Geometry: final body of the model. Coordinates: model frame, mm. A direction names the side the tool comes from. Coordinates: 2 decimals unless noted, no trailing zeros. Order: outer loops, then holes, each group sorted by start corner. A loop starts at its lowest first (then second) coordinate and runs counter-clockwise, first axis right, second up. Notation, with made-up numbers: M -28.75,46.5 L 10.25,46.5 A27 cw 10.25,64.5 Z; hole C -26.75,7 d2. An arc over 180 degrees is marked long. Use CSV: the item, a comma, the result in double quotes. Start each with the question number.
1. Material intervals for line 1 (X direction, y = -54.5, z = 7); line 2 (X direction, y = -17, z = 2.25); line 3 (Y direction, x = 32, z = 4.5), sorted ascending.
2. Section query D-D on x = 22. Return the cut outline in (y, z), and give its area (3 significant figures).
3. Section query C-C on z = 2.25. Return the cut outline in (x, y) (3 decimals), and give its area (3 significant figures).
4. Set-up query: faces 4 (the flat face through (-31.82, 37.9, 2.46)), 5 (the flat face through (65, 64, 15)), 6 (the flat face through (15, -24, 2)), 7 (the flat face through (-15, -23, 2)). Return all of +Z, -Z, +X, -X, +Y, -Y with unobstructed straight access to the full face (end or side cutting, diameter ignored); none if empty.
5. First-contact query: P1, Ø8, axis at y = 25.5, z = 7, coming from the +X side; P2, Ø1.5, axis at x = 38.5, z = 2, coming from the +Y side; P3, Ø2.5, axis at y = -23, z = 2.5, coming from the -X side. Flat tips, straight axial feed; report the tip coordinate or a pass-through.
6. Section query A-A on z = 9.25. Return the cut outline in (x, y) (3 decimals).
7. Section query B-B on y = 60.5. Return the cut outline in (x, z).
8. Pull-direction query (Y, two-part tool) for faces 1 (the cylindrical face through (0.061, 2.777, 2.535)), 2 (the flat face through (62, -59, 15)), 3 (the flat face through (42.415, 32.636, 2.465)); classes: pulls with the +Y half, pulls with the -Y half, needs draft (parallel to the pull), parting line crosses it, or undercut.
from build123d import *

# Parameters (mm, degrees)
F1_DEPTH = 5
F2_DEPTH = 15
F3_R     = 5


with BuildPart() as f1:
    # F0 (on Top) → F1 (new body)
    with BuildSketch(Plane.XY):
        with BuildLine():
            Line((-69.403826, 64.784578), (-15, -0.018286))
            Line((-15, -0.018286), (-15, -50.018286))
            Line((-15, -50.018286), (-65, -50.018286))
            ThreePointArc((-65, -50.018286), (-60.934136, -51.702422), (-59.25, -55.768286))
            ThreePointArc((-59.25, -55.768286), (-60.934136, -59.83415), (-65, -61.518286))
            Line((-65, -61.518286), (-15, -61.518286))
            Line((-15, -61.518286), (15, -61.518286))
            Line((15, -61.518286), (65, -61.518286))
            ThreePointArc((65, -61.518286), (59.25, -55.768286), (65, -50.018286))
            Line((65, -50.018286), (15, -50.018286))
            Line((15, -50.018286), (15, -0.018286))
            Line((15, -0.018286), (69.403826, 64.784578))
            ThreePointArc((69.403826, 64.784578), (61.302864, 64.077888), (60.596174, 72.17885))
            Line((60.596174, 72.17885), (0, 0))
            Line((0, 0), (-60.596174, 72.17885))
            ThreePointArc((-60.596174, 72.17885), (-59.597015, 70.449009), (-59.25, 68.481714))
            ThreePointArc((-59.25, 68.481714), (-63.032705, 63.078729), (-69.403826, 64.784578))
        make_face()
    extrude(amount=F1_DEPTH)

    # F0 (on Top) → F2 (join)
    with BuildSketch(Plane.XY):
        with BuildLine():
            Line((-65, -51.518286), (-65, -50.018286))
            ThreePointArc((-65, -50.018286), (-70.75, -55.768286), (-65, -61.518286))
            Line((-65, -61.518286), (-65, -60.018286))
            ThreePointArc((-65, -60.018286), (-69.25, -55.768286), (-65, -51.518286))
        make_face()
        with BuildLine():
            ThreePointArc((-59.25, -55.768286), (-60.934136, -51.702422), (-65, -50.018286))
            Line((-65, -50.018286), (-65, -51.518286))
            ThreePointArc((-65, -51.518286), (-61.994796, -52.763082), (-60.75, -55.768286))
            ThreePointArc((-60.75, -55.768286), (-61.994796, -58.77349), (-65, -60.018286))
            Line((-65, -60.018286), (-65, -61.518286))
            ThreePointArc((-65, -61.518286), (-60.934136, -59.83415), (-59.25, -55.768286))
        make_face()
        with BuildLine():
            ThreePointArc((65, -50.018286), (59.25, -55.768286), (65, -61.518286))
            Line((65, -61.518286), (65, -60.018286))
            ThreePointArc((65, -60.018286), (60.75, -55.768286), (65, -51.518286))
            Line((65, -51.518286), (65, -50.018286))
        make_face()
        with BuildLine():
            Line((65, -60.018286), (65, -61.518286))
            ThreePointArc((65, -61.518286), (69.065864, -59.83415), (70.75, -55.768286))
            ThreePointArc((70.75, -55.768286), (69.065864, -51.702422), (65, -50.018286))
            Line((65, -50.018286), (65, -51.518286))
            ThreePointArc((65, -51.518286), (68.005204, -52.763082), (69.25, -55.768286))
            ThreePointArc((69.25, -55.768286), (68.005204, -58.77349), (65, -60.018286))
        make_face()
        with BuildLine():
            Line((61.744998, 71.21438), (60.596174, 72.17885))
            ThreePointArc((60.596174, 72.17885), (61.302864, 64.077888), (69.403826, 64.784578))
            Line((69.403826, 64.784578), (68.255002, 65.749048))
            ThreePointArc((68.255002, 65.749048), (62.267334, 65.226712), (61.744998, 71.21438))
        make_face()
        with BuildLine():
            ThreePointArc((70.75, 68.481714), (66.967295, 73.884699), (60.596174, 72.17885))
            Line((60.596174, 72.17885), (61.744998, 71.21438))
            ThreePointArc((61.744998, 71.21438), (66.454088, 72.475225), (69.25, 68.481714))
            ThreePointArc((69.25, 68.481714), (68.993511, 67.027626), (68.255002, 65.749048))
            Line((68.255002, 65.749048), (69.403826, 64.784578))
            ThreePointArc((69.403826, 64.784578), (70.402985, 66.514419), (70.75, 68.481714))
        make_face()
        with BuildLine():
            ThreePointArc((-60.596174, 72.17885), (-68.697136, 72.88554), (-69.403826, 64.784578))
            Line((-69.403826, 64.784578), (-68.255002, 65.749048))
            ThreePointArc((-68.255002, 65.749048), (-67.732666, 71.736716), (-61.744998, 71.21438))
            Line((-61.744998, 71.21438), (-60.596174, 72.17885))
        make_face()
        with BuildLine():
            Line((-68.255002, 65.749048), (-69.403826, 64.784578))
            ThreePointArc((-69.403826, 64.784578), (-63.032705, 63.078729), (-59.25, 68.481714))
            ThreePointArc((-59.25, 68.481714), (-59.597015, 70.449009), (-60.596174, 72.17885))
            Line((-60.596174, 72.17885), (-61.744998, 71.21438))
            ThreePointArc((-61.744998, 71.21438), (-61.006489, 69.935802), (-60.75, 68.481714))
            ThreePointArc((-60.75, 68.481714), (-63.545912, 64.488203), (-68.255002, 65.749048))
        make_face()
    extrude(amount=F2_DEPTH)

    # F3
    f3_edges = [f1.edges().sort_by_distance(p)[0] for p in [
        (0, 0, 2.5),
        (-15, -0.018286, 2.5),
        (15, -0.018286, 2.5),
        (15, -50.018286, 2.5),
        (-15, -50.018286, 2.5),
    ]]
    fillet(f3_edges, radius=F3_R)


solid = f1.part
Results list:
1,line 1,"x = -70.61 to -69.06, -60.94 to -59.39, 59.39 to 60.94, 69.06 to 70.61"
1,line 2,"x = -15 to 15"
1,line 3,"y = -61.52 to -50.02, 20.23 to 38.12"
2,outline,"M -61.52,0 L -50.02,0 L -50.02,5 L -61.52,5 Z; M 8.32,0 L 26.21,0 L 26.21,5 L 8.32,5 Z"
2,area,"147 mm²"
3,outline,"M -69.404,64.785 L -16.171,1.376 A5 cw -15,-1.839 L -15,-45.018 A5 cw -20,-50.018 L -65,-50.018 A5.75 ccw -65,-61.518 L 65,-61.518 A5.75 ccw 65,-50.018 L 20,-50.018 A5 cw 15,-45.018 L 15,-1.839 A5 cw 16.171,1.376 L 69.404,64.785 A5.75 ccw 70.75,68.482 A5.75 ccw 60.596,72.179 L 3.829,4.561 A5 cw -3.829,4.561 L -60.596,72.179 A5.75 ccw Z; hole M -65,-51.518 A4.25 ccw long -60.75,-55.768 A4.25 ccw Z; hole M -61.745,71.214 A4.25 ccw long -60.75,68.482 A4.25 ccw Z; hole C 65,-55.768 d8.5; hole M 68.255,65.749 A4.25 ccw 69.25,68.482 A4.25 ccw long Z"
3,area,"5,050 mm²"
4,face 4,"+Z, -Z, +Y"
4,face 5,"+Z, +X, -X, +Y, -Y"
4,face 6,"+Z, -Z, +X"
4,face 7,"+Z, -Z, -X"
5,P1,"stops at x = 39.33"
5,P2,"stops at y = 46.75"
5,P3,"stops at x = -15"
6,outline,"C -65,-55.768 d11.5; M -60.596,72.179 A5.75 ccw long -59.25,68.482 A5.75 ccw Z; C 65,-55.768 d11.5; M 69.404,64.785 A5.75 ccw 70.75,68.482 A5.75 ccw long Z; hole M -65,-51.518 A4.25 ccw long -60.75,-55.768 A4.25 ccw Z; hole M -61.745,71.214 A4.25 ccw long -60.75,68.482 A4.25 ccw Z; hole C 65,-55.768 d8.5; hole M 68.255,65.749 A4.25 ccw 69.25,68.482 A4.25 ccw long Z"
7,outline,"M -65.81,0 L -50.79,0 L -50.79,5 L -65.81,5 Z; M 50.79,0 L 65.81,0 L 65.81,5 L 50.79,5 Z"
8,face 1,"pulls with the +Y half"
8,face 2,"needs draft"
8,face 3,"undercut"
